```python
from build123d import *

# Parameters (mm, degrees)
SKETCH1_R           = 3
BOSS_EXTRUDE1_DEPTH = 6.25
SKETCH2_R           = 6
BOSS_EXTRUDE2_DEPTH = 1.5


with BuildPart() as part:
    # Sketch1 → Boss-Extrude1 (new body)
    with BuildSketch(Plane.XY):
        Circle(SKETCH1_R)
    extrude(amount=BOSS_EXTRUDE1_DEPTH)

    # Sketch2 → Boss-Extrude2 (add)
    with BuildSketch(Plane.XY.offset(6.25)):
        Circle(SKETCH2_R)
    extrude(amount=BOSS_EXTRUDE2_DEPTH)

    # Sketch3 → Revolve1 (revolve)
    with BuildSketch(Plane(origin=(0, 0, 0), x_dir=(0, 0, -1), z_dir=(1, 0, 0))):
        with BuildLine():
            Line((-7.75, 6), (-7.75, 0.09036269))
            Line((-7.75, 0.09036269), (-10.197851923, 0.09036269))
            ThreePointArc((-10.197851923, 0.09036269), (-9.561675935, 3.288635355), (-7.75, 6))
        make_face()
    revolve(axis=Axis((0, 0, 6.25), (0, 0, -1)))


solid = part.part
```
For this review, take the finished solid that the model builds, in its own axes (mm). A direction names the side the tool comes from. Round coordinates to 2 decimals unless told otherwise and drop trailing zeros. Write each loop counter-clockwise with the first axis right and the second up, starting at its lowest first coordinate (ties: lowest second). Pieces come first, ordered by that corner, then holes. Notation, with made-up numbers: (13, 45) - (51, 45) arc R22 cw to (51, 84) - close; hole circle Ø10 at (-39.75, 14). An arc over 180 degrees is marked (long way). Answer as a JSON object with one key per item and string values.
1. For pin 1 Ø6 at (x, z) = (0, 2.5) entering from -Y; pin 2 Ø3 at (x, z) = (2, 6) entering from +Y; pin 3 Ø4 at (y, z) = (0.5, 5.5) entering from -X; pin 4 Ø5 at (y, z) = (3.5, 5) entering from -X, all flat-tipped, find the tip position at first contact; note any pin that passes through.
Response values:
{"pin 1": "stops at y = -3", "pin 2": "stops at y = 5.98", "pin 3": "stops at x = -6", "pin 4": "stops at x = -5.85"}
2. We need section B-B on z = 4.25. Give the boundary of the cut face in (x, y), then the cut area to 3 significant figures.
Response values:
{"outline": "circle Ø6 at (0, 0)", "area": "28.3 mm2"}
3. Tool access review of faces 1 (the face through (-3, 0, 3)), 2 (the face through (0, 0, 0)): name each direction out of +Z, -Z, +X, -X, +Y, -Y from which nothing blocks a thin tool from reaching the whole face with its end or side.
Response values:
{"face 1": "-Z", "face 2": "-Z, +X, -X, +Y, -Y"}
4. We need section A-A on z = 7. Give the boundary of the cut face in (x, y).
Response values:
{"outline": "circle Ø12 at (0, 0)"}
5. To check wall thickness, follow line 1 along X through (y, z) = (0, 8.6); line 2 along X through (y, z) = (0, 8.75); line 3 along Z through (x, y) = (-3.5, 4.75). State the ranges of each line that lie inside material, in increasing order.
Response values:
{"line 1": "x = -5.01 to -0.09, 0.09 to 5.01", "line 2": "x = -4.79 to -0.09, 0.09 to 4.79", "line 3": "z = 6.25 to 7.85"}
